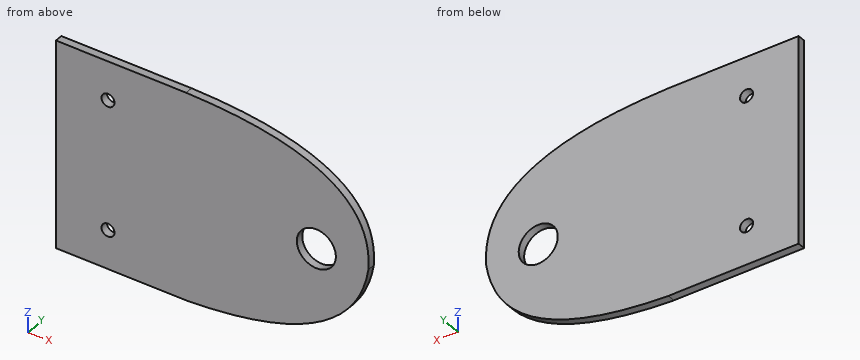
```python
from build123d import *

# Parameters (mm, degrees)
SKETCH1_R           = 2.5
SKETCH1_R_2         = 7.5
BOSS_EXTRUDE1_DEPTH = 3


with BuildPart() as part:
    # Sketch1 → Boss-Extrude1 (new body)
    with BuildSketch(Plane(origin=(0, 0, 0), x_dir=(1, 0, 0), z_dir=(0, 1, 0))):
        with BuildLine():
            Line((-100, 40), (-100, -40))
            Line((-100, -40), (-50, -40))
            add(Edge.make_bspline(
                [(-50, -40), (22.668262508, -38.849155335), (20, 0)],
                knots=[0, 0, 0, 0.942307838, 0.942307838, 0.942307838], degree=2))
            add(Edge.make_bspline(
                [(16.665092834, 11.057788243), (19.095873291, 5.971869908), (20, 0)],
                knots=[0.704383091, 0.704383091, 0.704383091, 0.839710595, 0.839710595, 0.839710595], degree=2))
            add(Edge.make_bspline(
                [(-50, 40), (4.01281886, 37.53012226), (16.665092834, 11.057788243)],
                knots=[0, 0, 0, 0.704383091, 0.704383091, 0.704383091], degree=2))
            Line((-50, 40), (-100, 40))
        make_face()
        with Locations(Location((-80, -25, 0), (0, 0, 270))):
            Circle(SKETCH1_R, mode=Mode.SUBTRACT)
        with Locations(Location((-80, 25, 0), (0, 0, 270))):
            Circle(SKETCH1_R, mode=Mode.SUBTRACT)
        with Locations(Location((0, 0, 0), (0, 0, 270))):
            Circle(SKETCH1_R_2, mode=Mode.SUBTRACT)
    extrude(amount=BOSS_EXTRUDE1_DEPTH)


solid = part.part
```
Input: part model. Units: mm. Frame: model coordinates. Coordinates: 2 decimals unless noted, no trailing zeros. Loops run counter-clockwise (first coordinate to the right, second up) from the corner with the lowest first, then second, coordinate; pieces in that order, holes last. Notation, with made-up numbers: M 85,64 L 108,64 A17 cw 108,90 Z; hole C 25,8 d6. An arc over 180 degrees is marked long. Use a Markdown table: item, result. Add a question column.
1) Section B-B, the plane y = 1.3. Give the number of separate pieces and of enclosed holes in the cut face, plus the area to 3 significant figures.
2) Section A-A, the plane x = -80. Return the cut outline in (y, z).
3) Pin query (flat end, axial travel): P1, Ø6, axis at x = 4, z = -31.5, coming from the -Y side. Return the tip coordinate at first contact, or that it passes through.
4) Line query: L1, parallel to X at y = 0.2, z = -2.5; L2, parallel to X at y = 2.1, z = 0; L3, parallel to Z at x = -18.5, y = 1.75. Output: solid intervals per line, ascending. Write a range as from..to.
Answer below:
| question | item | result |
|---|---|---|
| 1 | separate pieces | 1 |
| 1 | enclosed holes | 3 |
| 1 | area | 8,320 mm2 |
| 2 | outline | M 0,-40 L 3,-40 L 3,-27.5 L 0,-27.5 Z; M 0,-22.5 L 3,-22.5 L 3,22.5 L 0,22.5 Z; M 0,27.5 L 3,27.5 L 3,40 L 0,40 Z |
| 3 | P1 | through |
| 4 | L1 | -100..-7.07, 7.07..19.55 |
| 4 | L2 | -100..-7.5, 7.5..20 |
| 4 | L3 | -35.66..37.09 |
